Autodesk Inventor part; units mm, degrees
ref_plane "YZ Plane" through (0, 0, 0) normal (1, 0, 0) x (0, 1, 0)
ref_plane "XZ Plane" through (0, 0, 0) normal (0, 1, 0) x (-1, 0, 0)
ref_plane "XY Plane" through (0, 0, 0) normal (0, 0, 1) x (1, 0, 0)
sketch "Sketch1" plane through (0, 0, 0) normal (0, 1, 0) x (-1, 0, 0)
  line L0 (-0.4496, -29.3) -> (-0.4496, 0)
  line L1 (-41.2289, 0) -> (-41.2289, -29.3)
  circle A0 centre (-49.9386, -23.2) radius 1.05
  circle A1 centre (-50.9386, -9.98) radius 1.05
  circle A2 centre (-57.9386, -2.68) radius 1.05
  circle A3 centre (-64.9386, -9.98) radius 1.05
  circle A4 centre (-65.9386, -23.2) radius 1.05
  circle A5 centre (23.785, -2.5) radius 1.05
  circle A6 centre (8.735, -2.5) radius 1.05
  circle A7 centre (23.785, -17.6) radius 1.05
  circle A8 centre (8.735, -17.6) radius 1.05
  circle A9 centre (-25.6393, -7) radius 1.55
  circle A10 centre (-35.7793, -7) radius 1.55
  circle A11 centre (-25.6393, -22.3) radius 1.55
  circle A12 centre (-35.7793, -22.3) radius 1.55
  arc A13 (-67.0086, 0) -> (-68.0086, -1) centre (-67.0086, -1) ccw
  line L2 (-67.0086, 0) -> (25.33, 0)
  line L3 (-68.0086, -28.3) -> (-68.0086, -1)
  arc A14 (-68.0086, -28.3) -> (-67.0086, -29.3) centre (-67.0086, -28.3) ccw
  line L4 (-63.885, -29.3) -> (-67.0086, -29.3)
  arc A15 (-51.9921, -29.3) -> (-63.885, -29.3) centre (-57.9386, -30.1) ccw
  line L5 (10.3136, -29.3) -> (-51.9921, -29.3)
  arc A16 (22.2064, -29.3) -> (10.3136, -29.3) centre (16.26, -30.1) ccw
  line L6 (25.33, -29.3) -> (22.2064, -29.3)
  arc A17 (25.33, -29.3) -> (26.33, -28.3) centre (25.33, -28.3) ccw
  line L7 (26.33, -1) -> (26.33, -28.3)
  arc A18 (26.33, -1) -> (25.33, 0) centre (25.33, -1) ccw
  line L8 (-41.6786, -29.3) -> (-41.6786, 0)
  line L9 (-40.7793, 0) -> (-40.7793, -29.3)
  line L10 (-0.8993, -29.3) -> (-0.8993, 0)
  line L11 (0, 0) -> (0, -29.3)
  point P0 (0, 0)
extrude "Extrusion1" add sketch "Sketch1" against normal blind 1.5
properties part number "axis_22_bottom_frame"
The model under review builds one solid part; all positions refer to its coordinate system, in mm. Round coordinates to 2 decimals unless told otherwise and drop trailing zeros. Loops run counter-clockwise (first coordinate to the right, second up) from the corner with the lowest first, then second, coordinate; pieces in that order, holes last. Notation, with made-up numbers: M 82.25,34.25 L 106.25,34.25 A22 ccw 106.25,66.25 Z; hole C 86.5,12.25 d7. An arc over 180 degrees is marked long. Answer as CSV lines item,"result". Start each with the question number.
Item 1: Consider section C-C (z = -27.5). Write out the cut boundary in (x, y), then the cut area to 3 significant figures.
Item 2: Insertion check: P1, Ø3.5, axis at x = 35.78, z = -7, coming from the -Y side. The pin has a flat end and moves straight along its axis. Give the tip position at first contact, or say it passes through.
Item 3: Mouldability with a two-part tool opening along X and no side actions: class faces 1 (the face through (-8.507, -0.74, -3.525)), 2 (the face through (65, -1, -29.3)), 3 (the face through (68.009, -1, -15)) as released by +X, released by -X, zero draft, split by the parting line, or undercut.
Item 4: Consider section A-A (z = -9.98). Write out the cut boundary in (x, y), then the cut area to 3 significant figures.
Item 5: Consider section B-B (y = -0.75). State how many separate pieces and enclosed holes the cut face has, then the cut area to 3 significant figures.
Item 6: Wall thickness on line 1 (X direction, y = -1.25, z = -25); line 2 (X direction, y = -0.85, z = -3); line 3 (X direction, y = -0.8, z = -9.25): over which ranges is each line inside the solid? List them lowest first. Write a range as [from, to].
Item 7: Consider section D-D (x = 60). Write out the cut boundary in (y, z), then the cut area to 3 significant figures.
Answer:
1,outline,"M -26.33,-1.5 L -21.67,-1.5 L -21.67,0 L -26.33,0 Z; M -10.85,-1.5 L 52.53,-1.5 L 52.53,0 L -10.85,0 Z; M 63.35,-1.5 L 68.01,-1.5 L 68.01,0 L 63.35,0 Z"
1,area,"109 mm^2"
2,P1,"stops at y = -1.5"
3,face 1,"undercut"
3,face 2,"zero draft"
3,face 3,"released by +X"
4,outline,"M -26.33,-1.5 L 49.89,-1.5 L 49.89,0 L -26.33,0 Z; M 51.99,-1.5 L 63.89,-1.5 L 63.89,0 L 51.99,0 Z; M 65.99,-1.5 L 68.01,-1.5 L 68.01,0 L 65.99,0 Z"
4,area,"135 mm^2"
5,separate pieces,"1"
5,enclosed holes,"13"
5,area,"2,610 mm^2"
6,line 1,"x = [-26.33, -19.42], [-13.1, 54.78], [61.1, 68.01]"
6,line 2,"x = [-26.33, -24.71], [-22.86, -9.66], [-7.81, 56.94], [58.94, 68.01]"
6,line 3,"x = [-26.33, 50.18], [51.69, 64.18], [65.69, 68.01]"
7,outline,"M -1.5,-24.47 L 0,-24.47 L 0,0 L -1.5,0 Z"
7,area,"36.7 mm^2"
